Can you work these out from the drawing? Everything is in mm from the part's minimum corner. A direction names the side the tool comes from. Coordinates: 2 decimals unless noted, no trailing zeros. Order: outer loops, then holes, each group sorted by start corner. A loop starts at its lowest first (then second) coordinate and runs counter-clockwise, first axis right, second up. Notation, with made-up numbers: (-13, 37.5) - (11, 37.5) arc R20 cw to (11, 69.5) - close; hole circle Ø3 at (-1.75, 72). An arc over 180 degrees is marked (long way). Use a Markdown table: item, result. Add a question column.
(1) I want a section at B-B (y = 3.75). List the corners of the cut face in (x, z) for me.
(2) I want a section at C-C (x = 3.5). List the corners of the cut face in (y, z) for me.
(3) We'd pull the mould along X, two halves only. Please class the marked faces 1, 2 and 3: pulls with the +X half, pulls with the -X half, needs draft (parallel to the pull), parting line crosses it, or undercut.
(4) I want a section at D-D (y = 7). List the corners of the cut face in (x, z) for me, and give its area (3 significant figures).
(5) If I drill on L1, parallel to Z at x = 8.5, y = 1.5; L2, parallel to Z at x = 4.5, y = 4.5; L3, parallel to Y at x = 4.5, z = 16, over which ranges is the centre line in solid material (lowest first)? Write a range as [from, to].
(6) For pin 1 Ø1 at (x, y) = (2, 6.5) entering from -Z; pin 2 Ø0.9 at (y, z) = (5, 13.5) entering from +X; pin 3 Ø3.5 at (x, z) = (4, 16.5) entering from +Y; pin 4 Ø2 at (y, z) = (5, 17) entering from -X, each with a flat end and sliding along its axis, tell me the tip position at first contact or that it passes through.
(7) On a 3-axis mill with a long thin cutter (end or side, diameter ignored), from which of +Z, -Z, +X, -X, +Y, -Y can I reach the whole of each face in a straight line? I mean the marked faces 4, 5, 6, 7 and 8. Say none if no direction works.
(8) I want a section at A-A (z = 1). List the corners of the cut face in (x, y) for me, and give its area (3 significant figures).
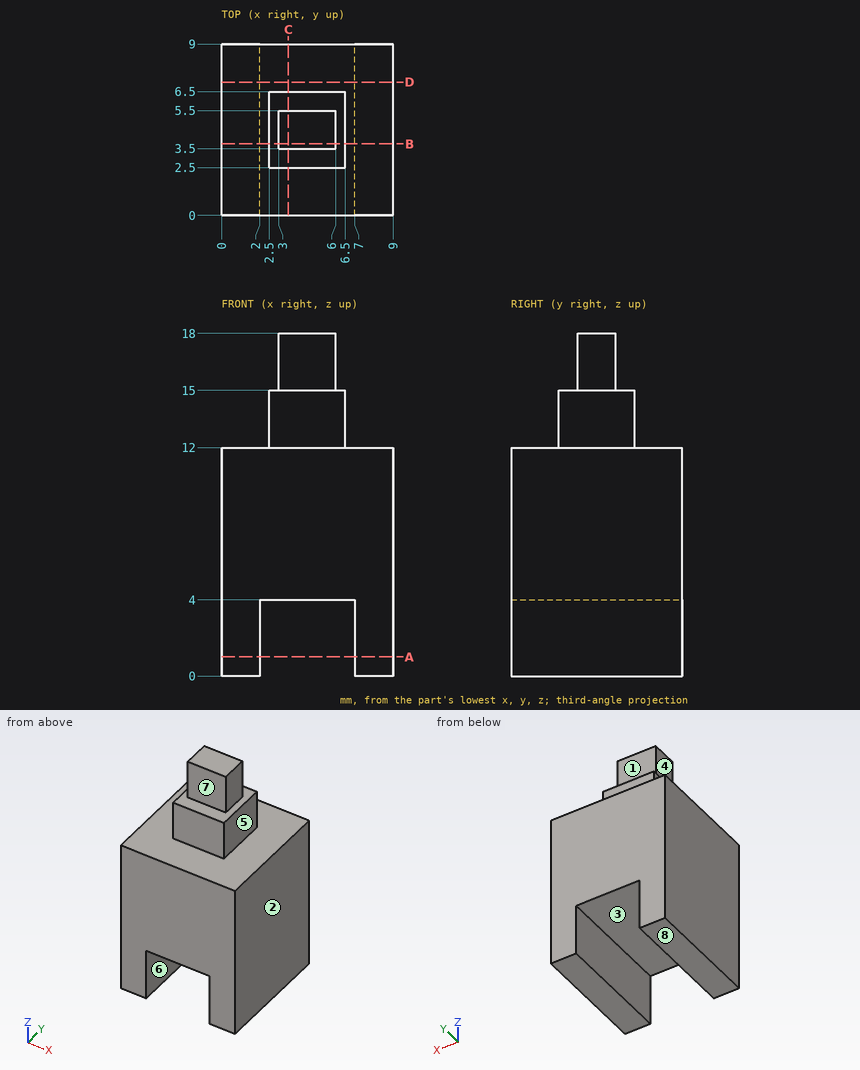
Answers follow:
| question | item | result |
|---|---|---|
| 1 | outline | (0, 0) - (2, 0) - (2, 4) - (7, 4) - (7, 0) - (9, 0) - (9, 12) - (6.5, 12) - (6.5, 15) - (6, 15) - (6, 18) - (3, 18) - (3, 15) - (2.5, 15) - (2.5, 12) - (0, 12) - close |
| 2 | outline | (0, 4) - (9, 4) - (9, 12) - (6.5, 12) - (6.5, 15) - (5.5, 15) - (5.5, 18) - (3.5, 18) - (3.5, 15) - (2.5, 15) - (2.5, 12) - (0, 12) - close |
| 3 | face 1 | needs draft |
| 3 | face 2 | pulls with the +X half |
| 3 | face 3 | undercut |
| 4 | outline | (0, 0) - (2, 0) - (2, 4) - (7, 4) - (7, 0) - (9, 0) - (9, 12) - (0, 12) - close |
| 4 | area | 88.0 mm² |
| 5 | L1 | z = [0, 12] |
| 5 | L2 | z = [4, 18] |
| 5 | L3 | y = [3.5, 5.5] |
| 6 | pin 1 | stops at z = 0 |
| 6 | pin 2 | stops at x = 6.5 |
| 6 | pin 3 | stops at y = 6.5 |
| 6 | pin 4 | stops at x = 3 |
| 7 | face 4 | +Z, -X, +Y, -Y |
| 7 | face 5 | +Z, +X, +Y, -Y |
| 7 | face 6 | -Z, +Y, -Y |
| 7 | face 7 | +Z, +X, -X, -Y |
| 7 | face 8 | -Z, +X, -X, +Y, -Y |
| 8 | outline | (0, 0) - (2, 0) - (2, 9) - (0, 9) - close; (7, 0) - (9, 0) - (9, 9) - (7, 9) - close |
| 8 | area | 36.0 mm² |
